Autodesk Inventor part; units mm, degrees
ref_plane "YZ Plane" through (0, 0, 0) normal (1, 0, 0) x (0, 1, 0)
ref_plane "XZ Plane" through (0, 0, 0) normal (0, 1, 0) x (-1, 0, 0)
ref_plane "XY Plane" through (0, 0, 0) normal (0, 0, 1) x (1, 0, 0)
sketch "Эскиз1" plane through (0, 0, 0) normal (0, 0, 1) x (1, 0, 0)
  line L0 (0, 0) -> (180, 0)
  line L1 (180, 0) -> (180, -30)
  line L2 (180, -30) -> (0, -30)
  line L3 (0, -30) -> (0, 0)
  line L4 (0, 0) -> (-6, 0)
  line L5 (-6, 0) -> (-6, -10)
  line L6 (-6, -10) -> (0, -10)
  line L7 (0, -10) -> (0, 0)
  line L8 (0, -20) -> (-6, -20)
  line L9 (-6, -20) -> (-6, -30)
  line L10 (-6, -30) -> (0, -30)
  line L11 (0, -30) -> (0, -20)
  line L12 (180, 0) -> (186, 0)
  line L13 (186, 0) -> (186, -10)
  line L14 (186, -10) -> (180, -10)
  line L15 (180, -10) -> (180, 0)
  line L16 (180, -30) -> (180, -20)
  line L17 (186, -20) -> (186, -30)
  line L18 (186, -30) -> (180, -30)
  line L19 (180, -20) -> (186, -20)
  dimension "d0" = 180
  dimension "d1" = 30
  dimension "d2" = 10
  dimension "d3" = 6
  dimension "d6" = 20
  dimension "d11" = 6
  dimension "d14" = 20
extrude "Выдавливание1" add sketch "Эскиз1" along normal blind 6
Read the model definition and answer for the solid it produces. Units are mm, in the model's axes. A direction names the side the tool comes from. Coordinates: 2 decimals unless noted, no trailing zeros. Loops run counter-clockwise (first coordinate to the right, second up) from the corner with the lowest first, then second, coordinate; pieces in that order, holes last.
Q1. This flat-tipped pin is pushed along its axis until it touches: pin 1 Ø1.8 at (y, z) = (-12.5, 2) entering from +X. Where does it stop, or does it pass through?
Q2. The mould has two halves that part along Y. Classify faces 4 (the face through (186, -5, 3)), 5 (the face through (89, 0, 3)), 6 (the face through (91, -30, 3)), 7 (the face through (-3, -20, 3)): +Y half, -Y half, draft (parallel to the pull), parting line (faces both ways), or undercut.
Q3. Consider probe 1 along X at (y, z) = (-19, 1.9). Determine where the line is inside the solid, lowest interval first.
Q4. Which of the six approach directions +Z, -Z, +X, -X, +Y, -Y give full straight-line access (tool end or side, diameter ignored) to faces 1 (the face through (0, -15, 3)), 2 (the face through (89, -15, 0)), 3 (the face through (180, -15, 3))?
Q5. The part is cut by section B-B on y = -15.75. Write down the section's boundary in (x, z).
Q6. The part is cut by section A-A on z = 4.75. Write down the section's boundary in (x, y).
Results below:
1. pin 1: stops at x = 180
2. face 4: draft
2. face 5: +Y half
2. face 6: -Y half
2. face 7: undercut
3. probe 1: x = 0 to 180
4. face 1: +Z, -Z, -X
4. face 2: -Z, +X, -X, +Y, -Y
4. face 3: +Z, -Z, +X
5. outline: (0, 0) - (180, 0) - (180, 6) - (0, 6) - close
6. outline: (-6, -30) - (186, -30) - (186, -20) - (180, -20) - (180, -10) - (186, -10) - (186, 0) - (-6, 0) - (-6, -10) - (0, -10) - (0, -20) - (-6, -20) - close
